Geometry check sheet. Reference: the model listing, model coordinates, mm. A direction names the side the tool comes from. Give positions to 0.01 mm unless a question says otherwise; leave off trailing zeros. Loops run counter-clockwise (first coordinate to the right, second up) from the corner with the lowest first, then second, coordinate; pieces in that order, holes last. Notation, with made-up numbers: (1, 23) -> (17, 23) arc R23 cw to (17, 36) -> close; hole circle Ø9 at (55.25, -22). An arc over 180 degrees is marked (long way). Answer as a JSON object with one key per item and string values.
Autodesk Inventor part; units mm, degrees
ref_plane "YZ Plane" through (0, 0, 0) normal (1, 0, 0) x (0, 1, 0)
ref_plane "XZ Plane" through (0, 0, 0) normal (0, 1, 0) x (-1, 0, 0)
ref_plane "XY Plane" through (0, 0, 0) normal (0, 0, 1) x (1, 0, 0)
sketch "Sketch1" plane through (0, 0, 0) normal (0, 0, 1) x (1, 0, 0)
  line L0 (-19.812, 0) -> (26.416, 0)
  line L1 (0, 36.83) -> (0, -16.51)
  line L2 (-16.51, -12.7) -> (16.51, -12.7)
  line L3 (16.51, -12.7) -> (16.51, 8.89)
  arc A0 (16.51, 8.89) -> (-16.51, 8.89) centre (0, 8.89) ccw
  line L4 (-16.51, 8.89) -> (-16.51, -12.7)
  dimension "d2" = 33.02
  dimension "d3" = 8.89
  dimension "d4" = 12.7
extrude "Extrusion1" add sketch "Sketch1" along normal blind 2.54
sketch "Sketch2" plane through (0, 0, 2.54) normal (0, 0, 1) x (1, 0, 0)
  line L0 (-16.51, -12.7) -> (-16.51, 8.89)
  line L1 (16.51, -12.7) -> (-16.51, -12.7)
  line L2 (16.51, 8.89) -> (16.51, -12.7)
  line L3 (-10.16, -12.7) -> (-10.16, 12.7)
  line L4 (-10.16, 12.7) -> (10.16, 12.7)
  line L5 (10.16, 12.7) -> (10.16, -12.7)
  dimension "d7" = 6.35
  dimension "d8" = 6.35
  dimension "d9" = 25.4
extrude "Extrusion2" add sketch "Sketch2" along normal blind 19
sketch "Sketch3" plane through (10.16, -12.7, 21.54) normal (1, 0, 0) x (0, 0, -1)
  line L0 (0, 25.4) -> (0, 0)
  line L1 (19, 25.4) -> (0, 25.4)
  point P0 (8.89, 16.51)
  dimension "d12" = 8.89
  dimension "d13" = 8.89
hole "Hole1" at (10.16, 3.81, 12.65) direction (-1, 0, 0) diameter 5 end through all
fillet "Fillet1" radius 2.54 3 edges at (10.16, 0, 2.54) (0, 12.7, 2.54) (-10.16, 0, 2.54)
sketch "Sketch6" plane through (-10.16, 12.7, 21.54) normal (0, 1, 0) x (1, 0, 0)
  line L0 (0, 16.46) -> (20.32, 16.46)
  line L1 (20.32, 16.46) -> (20.32, 0)
  line L2 (13.97, 14.555) -> (13.97, 10.6635)
  line L3 (13.97, 10.6635) -> (17.2354, 14.555)
  line L4 (17.2354, 14.555) -> (13.97, 14.555)
  dimension "d22" = 6.35
  dimension "d23" = 1.905
  dimension "d24" = 40
  dimension "d25" = 5.08
extrude "Extrusion3" cut sketch "Sketch6" against normal blind 12.5
sketch "Sketch7" plane through (-10.16, 12.7, 21.54) normal (0, 1, 0) x (1, 0, 0)
  line L0 (0, 16.46) -> (20.32, 16.46)
  line L1 (0, 16.46) -> (0, 0)
  circle A0 centre (8.89, 11.38) radius 1.905
  dimension "d28" = 8.89
  dimension "d29" = 5.08
  dimension "d30" = 3.81
extrude "Extrusion4" add sketch "Sketch7" along normal blind 2.54
sketch "Sketch8" plane through (-10.16, 12.7, 21.54) normal (0, 1, 0) x (1, 0, 0)
  line L0 (0, 16.46) -> (20.32, 16.46)
  line L1 (0, 16.46) -> (0, 0)
  line L2 (5.08, 14.428) -> (1.651, 14.428)
  line L3 (1.651, 14.428) -> (1.651, 12.396)
  line L4 (1.651, 12.396) -> (5.08, 12.396)
  line L5 (5.08, 12.396) -> (5.08, 14.428)
  dimension "d33" = 2.032
  dimension "d34" = 1.651
  dimension "d35" = 3.429
  dimension "d36" = 2.032
extrude "Extrusion5" cut sketch "Sketch8" against normal blind 2.54
properties part number "querylab"
1) Section check C-C on x = -1.27. Record the cut outline in (y, z) (3 decimals), plus the area to 3 significant figures.
Geometry check:
{"outline": "(-12.7, 0) -> (25.351, 0) -> (25.351, 2.54) -> (15.24, 2.54) arc R2.54 cw to (12.7, 5.08) -> (12.7, 8.255) -> (15.24, 8.255) -> (15.24, 12.065) -> (12.7, 12.065) -> (12.7, 21.54) -> (-12.7, 21.54) -> close; hole circle Ø5 at (3.81, 12.65)", "area": "571 mm2"}
2) Tool access check on faces 4 (the face through (-7, 11, 9.144)), 5 (the face through (0, 7, 0)), 6 (the face through (-1, 15.24, 10)), 7 (the face through (-10.884, 1.466, 3.304)), 8 (the face through (10.16, 0, 13)). Record the directions out of +Z, -Z, +X, -X, +Y, -Y that give a thin tool (end or side, any length) a straight path to the whole face; none if there is none.
Geometry check:
{"face 4": "+Y", "face 5": "-Z, +X, -X, +Y, -Y", "face 6": "+Z, +X, -X, +Y", "face 7": "+Z, -X, +Y, -Y", "face 8": "+Z, +X, +Y, -Y"}
3) Section check D-D on y = -0.5. Record the cut outline in (x, z).
Geometry check:
{"outline": "(-16.51, 0) -> (16.51, 0) -> (16.51, 2.54) -> (12.7, 2.54) arc R2.54 cw to (10.16, 5.08) -> (10.16, 21.54) -> (-10.16, 21.54) -> (-10.16, 5.08) arc R2.54 cw to (-12.7, 2.54) -> (-16.51, 2.54) -> close"}
4) Section check B-B on y = 3.81. Record the cut outline in (x, z) (3 decimals).
Geometry check:
{"outline": "(-16.51, 0) -> (16.51, 0) -> (16.51, 2.54) -> (12.7, 2.54) arc R2.54 cw to (10.16, 5.08) -> (10.16, 10.15) -> (4.42, 10.15) -> (7.075, 6.985) -> (3.81, 6.985) -> (3.81, 10.15) -> (-10.16, 10.15) -> (-10.16, 5.08) arc R2.54 cw to (-12.7, 2.54) -> (-16.51, 2.54) -> close; (-10.16, 15.15) -> (10.16, 15.15) -> (10.16, 21.54) -> (-10.16, 21.54) -> close"}
5) Material ranges on line 1 along Y through (x, z) = (-4, 12.65); line 2 along Z through (x, y) = (-2.5, 3.81); line 3 along Y through (x, z) = (0, 16), recorded low to high. Write a range as from..to.
Geometry check:
{"line 1": "y = -12.7..1.31, 6.31..12.7", "line 2": "z = 0..10.15, 15.15..21.54", "line 3": "y = -12.7..12.7"}
6) Depth check by flat-ended pin: P1, Ø6, axis at y = -1, z = 13, coming from the -X side; P2, Ø1.9, axis at x = -0.5, z = 9.5, coming from the +Y side; P3, Ø3.5, axis at x = 5.5, z = 9, coming from the +Y side. Enter the tip coordinate at first touch or a pass-through.
Geometry check:
{"P1": "stops at x = -10.16", "P2": "stops at y = 15.24", "P3": "stops at y = 12.7"}
7) Draft check along X on faces 1 (the face through (5, 7, 6.985)), 2 (the face through (16.51, -2, 1)), 3 (the face through (0, 0, 21.54)). Enter one of: pulls with the +X half, pulls with the -X half, needs draft (parallel to the pull), parting line crosses it, or undercut.
Geometry check:
{"face 1": "undercut", "face 2": "pulls with the +X half", "face 3": "needs draft"}
8) Section check A-A on z = 12.65. Record the cut outline in (x, y).
Geometry check:
{"outline": "(-10.16, -12.7) -> (10.16, -12.7) -> (10.16, 1.31) -> (-10.16, 1.31) -> close; (-10.16, 6.31) -> (10.16, 6.31) -> (10.16, 12.7) -> (-10.16, 12.7) -> close"}
